Check sheet for the drawn part. Datum: minimum x, y, z corner. Units: mm. A direction names the side the tool comes from. Round coordinates to 2 decimals unless told otherwise and drop trailing zeros. Write each loop counter-clockwise with the first axis right and the second up, starting at its lowest first coordinate (ties: lowest second). Pieces come first, ordered by that corner, then holes. Notation, with made-up numbers: (29, 7) -> (76, 7) arc R20 cw to (76, 33) -> close; hole circle Ø3 at (28.25, 40). An arc over 180 degrees is marked (long way). Use a Markdown table: item, result.
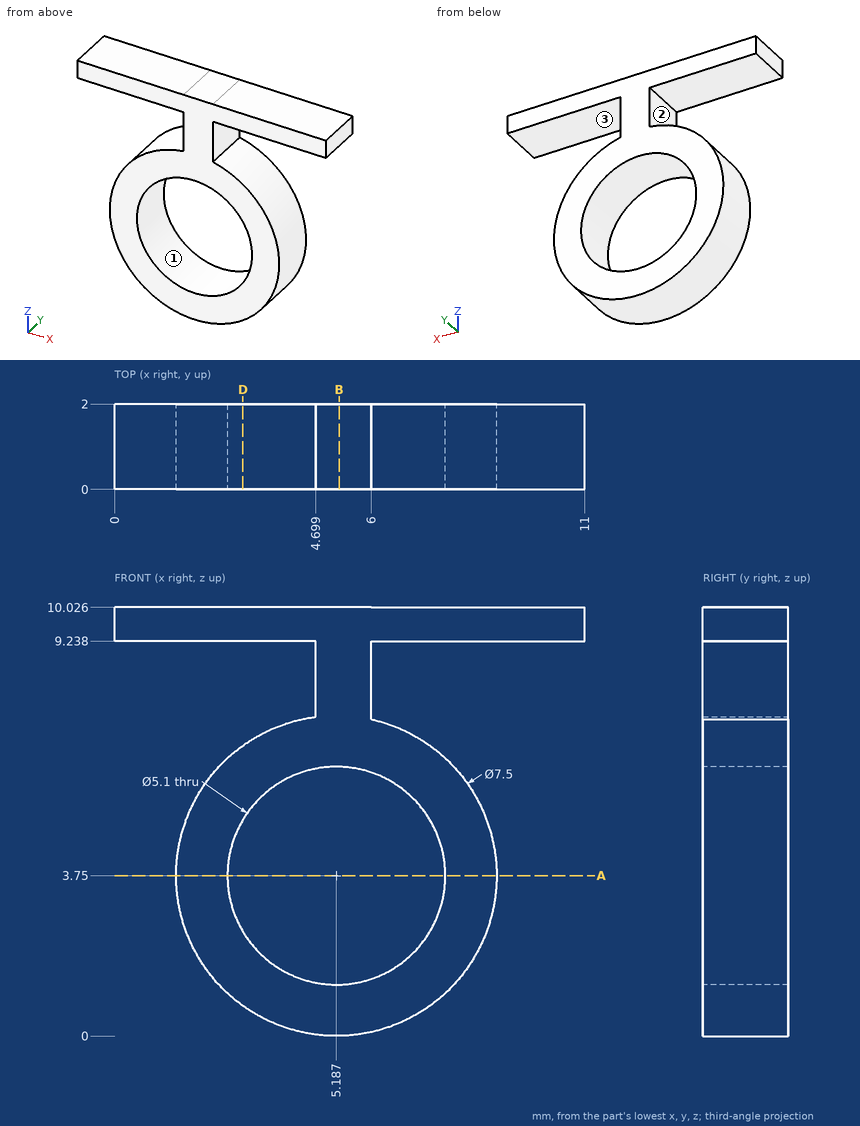
(1) Section check D-D on x = 3. Record the cut outline in (y, z) (1 decimal).
A:
| item | result |
|---|---|
| outline | (0, 0.7) -> (2, 0.7) -> (2, 2.4) -> (0, 2.4) -> close; (0, 5.1) -> (2, 5.1) -> (2, 6.8) -> (0, 6.8) -> close; (0, 9.2) -> (2, 9.2) -> (2, 10) -> (0, 10) -> close |
(2) Section check A-A on z = 3.75. Record the cut outline in (x, y).
A:
| item | result |
|---|---|
| outline | (1.44, 0) -> (2.64, 0) -> (2.64, 2) -> (1.44, 2) -> close; (7.74, 0) -> (8.94, 0) -> (8.94, 2) -> (7.74, 2) -> close |
(3) Thickness scan on line 1 (Z direction, x = 4.5, y = 1.15) (1 decimal); line 2 (Z direction, x = 6.5, y = 0.7) (1 decimal); line 3 (Z direction, x = 1, y = 1.7) (1 decimal). Record the ranges inside material, lowest first.
A:
| item | result |
|---|---|
| line 1 | z = 0.1 to 1.3, 6.2 to 7.4, 9.2 to 10 |
| line 2 | z = 0.2 to 1.6, 5.9 to 7.3, 9.2 to 10 |
| line 3 | z = 9.2 to 10 |
(4) Section check B-B on x = 5.25. Record the cut outline in (y, z) (1 decimal).
A:
| item | result |
|---|---|
| outline | (0, 0) -> (2, 0) -> (2, 1.2) -> (0, 1.2) -> close; (0, 6.3) -> (2, 6.3) -> (2, 10) -> (0, 10) -> close |
(5) Gauge pin test, flat ends, axial feed: pin 1 Ø0.6 at (x, y) = (2.5, 1) entering from -Z; pin 2 Ø0.5 at (y, z) = (1, 8) entering from -X. Record the tip position at first contact, or that the pin passes through.
A:
| item | result |
|---|---|
| pin 1 | stops at z = 0.86 |
| pin 2 | stops at x = 4.7 |
(6) Access from +Z, -Z, +X, -X, +Y, -Y to the whole of each face (thin tool, end or side, straight path). Record for the marked faces 1, 2 and 3.
A:
| item | result |
|---|---|
| face 1 | +Y, -Y |
| face 2 | -X, +Y, -Y |
| face 3 | +X, +Y, -Y |
